Design review of the part built by this model. Coordinates are the model's own, in mm. A direction names the side the tool comes from. Coordinates: 2 decimals unless noted, no trailing zeros. Loops run counter-clockwise (first coordinate to the right, second up) from the corner with the lowest first, then second, coordinate; pieces in that order, holes last. Notation, with made-up numbers: (-23, -0.5) - (3, -0.5) arc R20 ccw to (3, 22.5) - close; hole circle Ø2 at (-4, -27.5). An arc over 180 degrees is marked (long way). One line per question, with ' | ' between items.
from build123d import *

# Parameters (mm, degrees)
CROQUIS1_W    = 2
CROQUIS1_H    = 5
CHAFL_N2_SIZE = 0.5


# Read off the part's stored shape, not the designer's step: M14 Roscas Standard Taladro1
with BuildPart() as part:
    # Croquis1 → Revolución1 (revolve)
    with BuildSketch(Plane.XY):
        Polygon((0, 90), (0, 0), (2.998, 0), (2.998, 20), (3.998, 20), (3.998, 22.2), (3.8, 22.2), (3.8, 23), (3.998, 23), (3.998, 63), (7, 63), (7, 68), (7, 73), (5.9, 73), (5.9, 76), (7, 76), (7, 90), align=None)
        with Locations((8, 70.5)):
            Rectangle(CROQUIS1_W, CROQUIS1_H)
    revolve(axis=Axis((0, 0, 0), (0, 1, 0)))

    # M14 Roscas Standard Taladro1 outline → M14 Roscas Standard Taladro1 (revolve, cut)
    with BuildSketch(Plane.XY):
        Polygon((7, 90), (5.8985, 90), (7, 88.8985), align=None)
    revolve(axis=Axis((0, 0, 0), (0, 1, 0)), mode=Mode.SUBTRACT)

    # Chaflán2
    chafl_n2_edges = [part.edges().sort_by_distance(p)[0] for p in [
        (-3.998, 20, 0),
        (-2.998, 0, 0),
    ]]
    chamfer(chafl_n2_edges, length=CHAFL_N2_SIZE)


solid = part.part
Q1. Take a section at B-B (y = 54.5). Give the boundary of the cut face in (x, z).
Returned:
outline: circle Ø8 at (0, 0)
Q2. For pin 1 (5 mm diameter, centred on x = -5.5, z = 1.5, fed in from -Y); pin 2 (4 mm diameter, centred on x = 7, y = 50.5, fed in from +Z); pin 3 (5 mm diameter, centred on y = 37.5, z = 0.5, fed in from +X); pin 4 (4 mm diameter, centred on x = 0, y = 49.5, fed in from +Z), all flat-tipped, find the tip position at first contact; note any pin that passes through.
Returned:
pin 1: stops at y = 20 | pin 2: passes through | pin 3: stops at x = 4 | pin 4: stops at z = 4
Q3. Draft analysis for pull direction Y (two halves, no side actions). For faces 1 (the flat face through (2, 73, 6)), 2 (the flat face through (-3, 63, 3)), 3 (the cylindrical face through (6.466, 65.535, 2.681)), state which applies: +Y half, -Y half, draft (parallel to the pull), parting line (faces both ways), or undercut.
Returned:
face 1: undercut | face 2: -Y half | face 3: draft
Q4. Take a section at A-A (y = 71). Give the boundary of the cut face in (x, z).
Returned:
outline: circle Ø18 at (0, 0)
Q5. Tool access review of faces 4 (the cylindrical face through (-0.52, 21.362, -3.964)), 5 (the cylindrical face through (6.466, 82.54, 2.681)), 6 (the cylindrical face through (-5.894, 74.521, -0.259)): name each direction out of +Z, -Z, +X, -X, +Y, -Y from which nothing blocks a thin tool from reaching the whole face with its end or side.
Returned:
face 4: -Y | face 5: +Y | face 6: none
Q6. To check wall thickness, follow line 1 along Y through (x, z) = (1.5, 8); line 2 along X through (y, z) = (80, 3.75); line 3 along Y through (x, z) = (6, -1). State the ranges of each line that lie inside material, in increasing order.
Returned:
line 1: y = 68 to 73 | line 2: x = -5.91 to 5.91 | line 3: y = 63 to 73, 76 to 89.82
